from build123d import *

# Parameters (mm, degrees)
SKETCH1_R               = 3
BOSS_EXTRUDE1_DEPTH     = 53
FILLET1_R               = 0.25
SKETCH2_R               = 0.75
CUT_EXTRUDE1_DEPTH      = 4.0000001
CUT_EXTRUDE1_DEPTH_BACK = 4.0000001
SKETCH4_W               = 15
SKETCH4_H               = 5
CUT_EXTRUDE2_DEPTH      = 53


with BuildPart() as part:
    # Sketch1 → Boss-Extrude1 (new body)
    with BuildSketch(Plane.XY):
        Circle(SKETCH1_R)
    extrude(amount=BOSS_EXTRUDE1_DEPTH)

    # Fillet1
    fillet1_edges = [part.edges().sort_by_distance(p)[0] for p in [
        (-3, 0, 0),
        (-3, 0, 53),
    ]]
    fillet(fillet1_edges, radius=FILLET1_R)

    # Sketch2 → Cut-Extrude1 (cut, two sides)
    with BuildSketch(Plane(origin=(0, 0, 0), x_dir=(0, 0, -1), z_dir=(1, 0, 0))) as cut_extrude1_sk:
        with Locations((-2.5, 0)):
            Circle(SKETCH2_R)
    extrude(amount=CUT_EXTRUDE1_DEPTH, mode=Mode.SUBTRACT)
    extrude(cut_extrude1_sk.sketch, amount=-CUT_EXTRUDE1_DEPTH_BACK, mode=Mode.SUBTRACT)

    # Sketch4 → Cut-Extrude2 (cut)
    with BuildSketch(Plane(origin=(0, 2.25, 0), x_dir=(1, 0, 0), z_dir=(0, 1, 0))):
        with Locations((0.79883006, -50.5)):
            Rectangle(SKETCH4_W, SKETCH4_H)
    extrude(amount=CUT_EXTRUDE2_DEPTH, mode=Mode.SUBTRACT)


solid = part.part
Verification items for the finished model (mm, model axes). A direction names the side the tool comes from. Round coordinates to 2 decimals unless told otherwise and drop trailing zeros. Loops run counter-clockwise (first coordinate to the right, second up) from the corner with the lowest first, then second, coordinate; pieces in that order, holes last. Notation, with made-up numbers: (24, -30.5) - (83, -30.5) arc R9 ccw to (83, -16.5) - close; hole circle Ø5 at (50, 83.25). An arc over 180 degrees is marked (long way). Use a Markdown table: item, result. Add a question column.
1. Section check B-B, the plane z = 25. Record the boundary of the cut face in (x, y), plus the area to 3 significant figures.
2. Section check A-A, the plane z = 2.5. Record the boundary of the cut face in (x, y), plus the area to 3 significant figures.
3. Access from +Z, -Z, +X, -X, +Y, -Y to the whole of each face (thin tool, end or side, straight path). Record for faces 1 (the face through (0, 0, 0)), 2 (the face through (0, 2.25, 50)).
4. Gauge pin test, flat ends, axial feed: pin 1 (1.5 mm diameter, centred on y = 2, z = 9, fed in from -X); pin 2 (1 mm diameter, centred on x = 1.5, y = -1.5, fed in from -Z); pin 3 (1 mm diameter, centred on x = -1, z = 34.5, fed in from +Y); pin 4 (1.2 mm diameter, centred on x = 0, z = 51.5, fed in from +Y). Record the tip position at first contact, or that the pin passes through.
5. Thickness scan on probe 1 along Z at (x, y) = (-0.7, 0); probe 2 along Y at (x, z) = (2.25, 25.5); probe 3 along Z at (x, y) = (1.75, -0.5). Record the ranges inside material, lowest first. Write a range as [from, to].
Checks:
| question | item | result |
|---|---|---|
| 1 | outline | circle Ø6 at (0, 0) |
| 1 | area | 28.3 mm^2 |
| 2 | outline | (-2.9, -0.75) arc R3 ccw to (2.9, -0.75) - close; (-2.9, 0.75) - (2.9, 0.75) arc R3 ccw to start |
| 2 | area | 19.4 mm^2 |
| 3 | face 1 | -Z, +X, -X, +Y, -Y |
| 3 | face 2 | +Z, +X, -X, +Y |
| 4 | pin 1 | stops at x = -2.73 |
| 4 | pin 2 | stops at z = 0 |
| 4 | pin 3 | stops at y = 2.96 |
| 4 | pin 4 | stops at y = 2.25 |
| 5 | probe 1 | z = [0, 1.75], [3.25, 53] |
| 5 | probe 2 | y = [-1.98, 1.98] |
| 5 | probe 3 | z = [0, 1.94], [3.06, 53] |
